Work out the finished part from the listing and answer in its coordinate system (mm). A direction names the side the tool comes from. Coordinates: 2 decimals unless noted, no trailing zeros. Write each loop counter-clockwise with the first axis right and the second up, starting at its lowest first coordinate (ties: lowest second). Pieces come first, ordered by that corner, then holes. Notation, with made-up numbers: M -17,-31 L -3,-31 A16 cw -3,-24 Z; hole C -14.5,70.25 d7. An arc over 180 degrees is marked long. Answer as CSV lines item,"result". Start each with the question number.
(1) A cutting plane is placed at A-A on z = 4.5. Give the vertices of the cut face in (x, y).
(2) Find the intervals of material crossed by L1, parallel to X at y = 10.5, z = 4.5; L2, parallel to Y at x = 18, z = 5.75; L3, parallel to X at y = 21.5, z = 6.5, in increasing order. Write a range as [from, to].
(3) A cutting plane is placed at B-B on x = 6.5. Give the vertices of the cut face in (y, z), then the cut area to 3 significant figures.
(4) Flat-ended cylindrical pins translate along their axes: P1, Ø1.6, axis at x = 1, y = 17.5, coming from the +Z side; P2, Ø0.6, axis at x = 45.5, y = 26, coming from the +Z side; P3, Ø12, axis at x = 23, y = 17, coming from the +Z side. Find the tip coordinate at first contact, or state that the pin passes through.
(5) A cutting plane is placed at C-C on y = 26. Give the vertices of the cut face in (x, z).
(6) The mould has two halves that part along Y. Classify faces 1 (the flat face through (0, 14, 3)), 2 (the flat face through (2, 14, 5)): released by +Y, released by -Y, zero draft, split by the parting line, or undercut.
(7) A cutting plane is placed at D-D on y = 22.5. Give the vertices of the cut face in (x, z).
(8) For faces 3 (the flat face through (3.2, 14, 5)), 4 (the flat face through (1, 7, 6)), 5 (the flat face through (24, 14, 0)), determine the directions among +Z, -Z, +X, -X, +Y, -Y from which every point of the face is accessible in a straight line to the end or side of a thin tool.
from build123d import *

# Parameters (mm, degrees)
SKETCH_W        = 48
SKETCH_H        = 28
PAD_DEPTH       = 8
SKETCH001_W     = 41.6
SKETCH001_H     = 21.6
POCKET_DEPTH    = 5
SKETCH002_W     = 4.279463
SKETCH002_H     = 10
POCKET001_DEPTH = 2.8
SKETCH003_W     = 2
SKETCH003_H     = 18
PAD001_DEPTH    = 1
SKETCH004_W     = 14.332329
SKETCH004_H     = 4
POCKET002_DEPTH = 2
SKETCH005_R     = 1
POCKET003_DEPTH = 3


with BuildPart() as part:
    # Sketch → Pad (new body)
    with BuildSketch(Plane.XY):
        with Locations((24, 14)):
            Rectangle(SKETCH_W, SKETCH_H)
    extrude(amount=PAD_DEPTH)

    # Sketch001 → Pocket (cut)
    with BuildSketch(Plane.XY.offset(8)):
        with Locations((24, 14)):
            Rectangle(SKETCH001_W, SKETCH001_H)
    extrude(amount=-POCKET_DEPTH, mode=Mode.SUBTRACT)

    # Sketch002 → Pocket001 (cut)
    with BuildSketch(Plane.XY.offset(8)):
        with Locations((2.139731, 14)):
            Rectangle(SKETCH002_W, SKETCH002_H)
    extrude(amount=-POCKET001_DEPTH, mode=Mode.SUBTRACT)

    # Sketch003 → Pad001 (new body)
    with BuildSketch(Plane.XY.offset(3)):
        with Locations((6.978305, 14)):
            Rectangle(SKETCH003_W, SKETCH003_H)
        with Locations((38.519785, 14)):
            Rectangle(SKETCH003_W, SKETCH003_H)
    extrude(amount=PAD001_DEPTH)

    # Sketch004 → Pocket002 (cut)
    with BuildSketch(Plane(origin=(0, 0, 0), x_dir=(0, -1, 0), z_dir=(-1, 0, 0))):
        with Locations((-14.166164, 6)):
            Rectangle(SKETCH004_W, SKETCH004_H)
    extrude(amount=-POCKET002_DEPTH, mode=Mode.SUBTRACT)

    # Sketch005 → Pocket003 (cut)
    with BuildSketch(Plane.XY.offset(8)):
        with Locations((2, 26)):
            Circle(SKETCH005_R)
        with Locations((2, 1.768416)):
            Circle(SKETCH005_R)
        with Locations((45.92067, 1.768416)):
            Circle(SKETCH005_R)
        with Locations((45.92067, 26)):
            Circle(SKETCH005_R)
    extrude(amount=-POCKET003_DEPTH, mode=Mode.SUBTRACT)


solid = part.part
Here are the results:
1,outline,"M 0,0 L 48,0 L 48,28 L 0,28 L 0,21.33 L 2,21.33 L 2,7 L 0,7 Z; hole M 3.2,3.2 L 44.8,3.2 L 44.8,24.8 L 3.2,24.8 Z"
2,L1,"x = [2, 3.2], [44.8, 48]"
2,L2,"y = [0, 3.2], [24.8, 28]"
2,L3,"x = [0, 3.2], [44.8, 48]"
3,outline,"M 0,0 L 28,0 L 28,8 L 24.8,8 L 24.8,3 L 23,3 L 23,4 L 5,4 L 5,3 L 3.2,3 L 3.2,8 L 0,8 Z"
3,area,"134 mm^2"
4,P1,"stops at z = 4"
4,P2,"stops at z = 5"
4,P3,"stops at z = 3"
5,outline,"M 0,0 L 48,0 L 48,8 L 46.92,8 L 46.92,5 L 44.92,5 L 44.92,8 L 3,8 L 3,5 L 1,5 L 1,8 L 0,8 Z"
6,face 1,"zero draft"
6,face 2,"undercut"
7,outline,"M 0,0 L 48,0 L 48,8 L 44.8,8 L 44.8,3 L 39.52,3 L 39.52,4 L 37.52,4 L 37.52,3 L 7.98,3 L 7.98,4 L 5.98,4 L 5.98,3 L 3.2,3 L 3.2,8 L 0,8 Z"
8,face 3,"+Z"
8,face 4,"+Z, -X"
8,face 5,"-Z, +X, -X, +Y, -Y"
